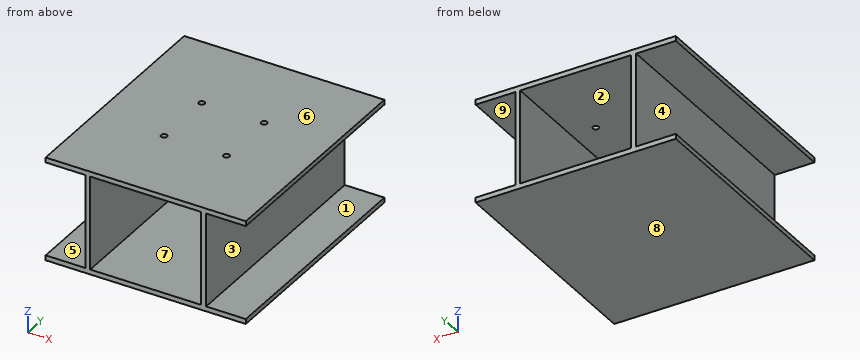
```python
from build123d import *

# Parameters (mm, degrees)
F0_W     = 320.675
F0_H     = 368.3
F1_DEPTH = 166.06266
F3_D     = 9.525
F3_DEPTH = 38.1
F4_W     = 63.5
F4_H     = 150.18766
F4_W_2   = 177.8
F5_DEPTH = 368.301


with BuildPart() as f1:
    # F0 (on Top) → F1 (new body)
    with BuildSketch(Plane.XY):
        with Locations((-0.724893, 21.601411)):
            Rectangle(F0_W, F0_H)
    extrude(amount=F1_DEPTH)

    # F3
    with Locations(Plane.XY.offset(166.06266)):
        with Locations((-50.724693, 69.373731), (49.275107, 69.373731), (49.275107, -30.626069), (-50.724693, -30.626069)):
            Hole(F3_D / 2, depth=F3_DEPTH)

    # F4 (on face) → F5 (cut, through all)
    with BuildSketch(Plane.XZ.offset(162.548589)):
        with Locations((-129.312393, 83.03133)):
            Rectangle(F4_W, F4_H)
        with Locations((127.862607, 83.03133)):
            Rectangle(F4_W, F4_H)
        with Locations((-0.724893, 83.03133)):
            Rectangle(F4_W_2, F4_H)
    extrude(amount=-F5_DEPTH, mode=Mode.SUBTRACT)


solid = f1.part
```
Model file for the job. Use its own axes, mm. Face numbers are marked on the shaded views. A direction names the side the tool comes from. Give positions to 0.01 mm unless a question says otherwise; leave off trailing zeros. Loops run counter-clockwise (first coordinate to the right, second up) from the corner with the lowest first, then second, coordinate; pieces in that order, holes last. Notation, with made-up numbers: M 65.25,-29 L 76.25,-29 A29 ccw 76.25,5 Z; hole C 79.5,30 d1. An arc over 180 degrees is marked long. Use one line per item in the form item = value.
Item 1: Slice it at C-C on x = -110.5. List the corners of the cut face in (y, z).
Filled in:
outline = M -162.55,0 L 205.75,0 L 205.75,7.94 L -162.55,7.94 Z; M -162.55,158.13 L 205.75,158.13 L 205.75,166.06 L -162.55,166.06 Z
Item 2: Slice it at B-B on y = 151. List the corners of the cut face in (x, z).
Filled in:
outline = M -161.06,0 L 159.61,0 L 159.61,7.94 L 96.11,7.94 L 96.11,158.13 L 159.61,158.13 L 159.61,166.06 L -161.06,166.06 L -161.06,158.13 L -97.56,158.13 L -97.56,7.94 L -161.06,7.94 Z; hole M -89.62,7.94 L 88.18,7.94 L 88.18,158.13 L -89.62,158.13 Z
Item 3: Flat gauge pins, fed straight in: pin 1 Ø1 at (y, z) = (127.5, 54) entering from +X; pin 2 Ø8.5 at (x, y) = (-50.72, -30.63) entering from +Z; pin 3 Ø8 at (y, z) = (-83.5, 134.5) entering from -X. Where does each tip first touch, or does it go through?
Filled in:
pin_1 = 96.11
pin_2 = 7.94
pin_3 = -97.56
Item 4: Two-plate mould, pull along X, no slides. Class the marked faces 1, 2, 3 and 4: released by +X, released by -X, zero draft, split by the parting line, or undercut.
Filled in:
face_1 = zero draft
face_2 = undercut
face_3 = released by +X
face_4 = released by -X
Item 5: Slice it at A-A on z = 140.5. List the corners of the cut face in (x, y), and give its area (3 significant figures).
Filled in:
outline = M -97.56,-162.55 L -89.62,-162.55 L -89.62,205.75 L -97.56,205.75 Z; M 88.18,-162.55 L 96.11,-162.55 L 96.11,205.75 L 88.18,205.75 Z
area = 5,850 mm^2
Item 6: Drill centre lines: L1, parallel to X at y = 45.5, z = 17; L2, parallel to Z at x = -44.5, y = 86. Where is each one in solid material? Low to high.
Filled in:
L1 = -97.56 to -89.62, 88.18 to 96.11
L2 = 0 to 7.94, 158.13 to 166.06
Item 7: Which spindle directions (+Z, -Z, +X, -X, +Y, -Y) get a long thin tool onto all of the face, cutting with end or side? Do the marked faces 5, 6, 7, 8 and 9. Say none if no direction does.
Filled in:
face_5 = -X, +Y, -Y
face_6 = +Z, +X, -X, +Y, -Y
face_7 = +Y, -Y
face_8 = -Z, +X, -X, +Y, -Y
face_9 = +X, +Y, -Y
